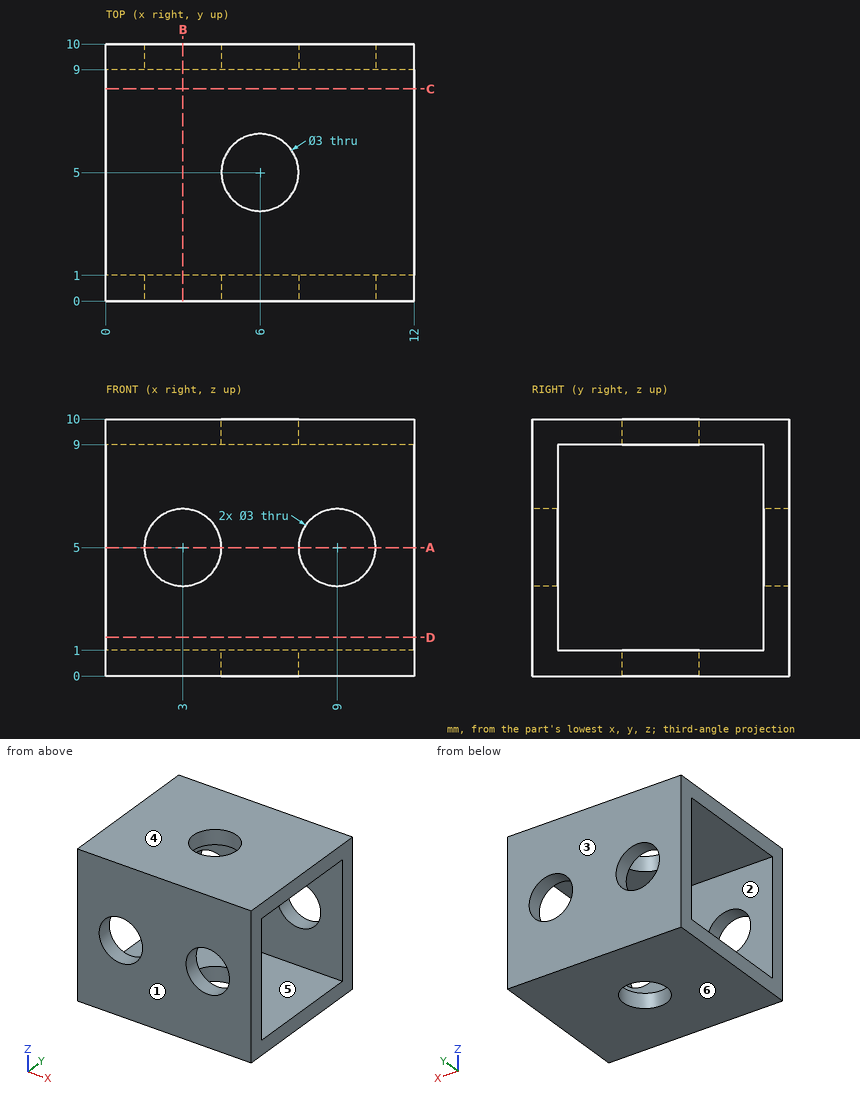
Can you work these out from the drawing? Everything is in mm from the part's minimum corner. A direction names the side the tool comes from. Round coordinates to 2 decimals unless told otherwise and drop trailing zeros. Write each loop counter-clockwise with the first axis right and the second up, starting at its lowest first coordinate (ties: lowest second). Pieces come first, ordered by that corner, then holes. Notation, with made-up numbers: (-37.75, 45.25) - (-8.75, 45.25) arc R18 cw to (-8.75, 54.25) - close; hole circle Ø3 at (48, 52). An arc over 180 degrees is marked (long way). Use a Markdown table: item, result.
Q1. Thinking about a two-plate mould opening in Y: for the marked faces 1, 2, 3 and 4, which applies, released by +Y, released by -Y, zero draft, split by the parting line, or undercut?
Output values:
| item | result |
|---|---|
| face 1 | released by -Y |
| face 2 | undercut |
| face 3 | released by +Y |
| face 4 | zero draft |
Q2. I want a section at B-B (x = 3). List the corners of the cut face in (y, z) for me.
Output values:
| item | result |
|---|---|
| outline | (0, 0) - (10, 0) - (10, 3.5) - (9, 3.5) - (9, 1) - (1, 1) - (1, 3.5) - (0, 3.5) - close; (0, 6.5) - (1, 6.5) - (1, 9) - (9, 9) - (9, 6.5) - (10, 6.5) - (10, 10) - (0, 10) - close |
Q3. I want a section at A-A (z = 5). List the corners of the cut face in (x, y) for me, plus the area to 3 significant figures.
Output values:
| item | result |
|---|---|
| outline | (0, 0) - (1.5, 0) - (1.5, 1) - (0, 1) - close; (0, 9) - (1.5, 9) - (1.5, 10) - (0, 10) - close; (4.5, 0) - (7.5, 0) - (7.5, 1) - (4.5, 1) - close; (4.5, 9) - (7.5, 9) - (7.5, 10) - (4.5, 10) - close; (10.5, 0) - (12, 0) - (12, 1) - (10.5, 1) - close; (10.5, 9) - (12, 9) - (12, 10) - (10.5, 10) - close |
| area | 12.0 mm2 |
Q4. For the marked faces 5 and 6, which set-ups out of +Z, -Z, +X, -X, +Y, -Y let a thin tool reach every point of the face, with its end or its side?
Output values:
| item | result |
|---|---|
| face 5 | +X, -X |
| face 6 | -Z, +X, -X, +Y, -Y |
Q5. For pin 1 (3.5 mm diameter, centred on x = 9, z = 5, fed in from -Y), with a flat end and sliding along its axis, tell me the tip position at first contact or that it passes through.
Output values:
| item | result |
|---|---|
| pin 1 | y = 0 |
Q6. I want a section at C-C (y = 8.25). List the corners of the cut face in (x, z) for me.
Output values:
| item | result |
|---|---|
| outline | (0, 0) - (12, 0) - (12, 1) - (0, 1) - close; (0, 9) - (12, 9) - (12, 10) - (0, 10) - close |
Q7. Please list where these lines run through material, in increasing order: L1, parallel to X at y = 0.2, z = 5; L2, parallel to Z at x = 1.5, y = 4.25; L3, parallel to Z at x = 3, y = 0.7.
Output values:
| item | result |
|---|---|
| L1 | 0 to 1.5, 4.5 to 7.5, 10.5 to 12 |
| L2 | 0 to 1, 9 to 10 |
| L3 | 0 to 3.5, 6.5 to 10 |
